from build123d import *

# Parameters (mm, degrees)
F0_R     = 5
F2_DEPTH = 3
F0_R_2   = 1.25
F3_DEPTH = 6
F4_DEPTH = 2


with BuildPart() as f2:
    # F0 (on Top) → F2 (new body)
    with BuildSketch(Plane.XY):
        with BuildLine():
            Line((-6.914658343, 3.5), (-14.0712472795, 3.5))
            ThreePointArc((-14.0712472795, 3.5), (-14.5, 0), (-14.0712472795, -3.5))
            Line((-14.0712472795, -3.5), (-6.914658343, -3.5))
            ThreePointArc((-6.914658343, -3.5), (-7.75, 0), (-6.914658343, 3.5))
        make_face()
        with BuildLine():
            ThreePointArc((7.75, 0), (7.5382724201, 1.7991522784), (6.914658343, 3.5))
            ThreePointArc((6.914658343, 3.5), (0, 7.75), (-6.914658343, 3.5))
            ThreePointArc((-6.914658343, 3.5), (-7.75, 0), (-6.914658343, -3.5))
            ThreePointArc((-6.914658343, -3.5), (0, -7.75), (6.914658343, -3.5))
            ThreePointArc((6.914658343, -3.5), (7.5382724201, -1.7991522784), (7.75, 0))
        make_face()
        Circle(F0_R, mode=Mode.SUBTRACT)
        with BuildLine():
            ThreePointArc((14.0712472795, -3.5), (14.3924126809, -1.7630817405), (14.5, 0))
            ThreePointArc((14.5, 0), (14.3924126809, 1.7630817405), (14.0712472795, 3.5))
            Line((14.0712472795, 3.5), (6.914658343, 3.5))
            ThreePointArc((6.914658343, 3.5), (7.5382724201, 1.7991522784), (7.75, 0))
            ThreePointArc((7.75, 0), (7.5382724201, -1.7991522784), (6.914658343, -3.5))
            Line((6.914658343, -3.5), (14.0712472795, -3.5))
        make_face()
    extrude(amount=F2_DEPTH)

    # F0 (on Top) → F3 (join)
    with BuildSketch(Plane.XY):
        with BuildLine():
            Line((6.914658343, 3.5), (14.0712472795, 3.5))
            ThreePointArc((14.0712472795, 3.5), (0, 14.5), (-14.0712472795, 3.5))
            Line((-14.0712472795, 3.5), (-6.914658343, 3.5))
            ThreePointArc((-6.914658343, 3.5), (0, 7.75), (6.914658343, 3.5))
        make_face()
        with Locations((-7.9549512883, 7.9549512883)):
            Circle(F0_R_2, mode=Mode.SUBTRACT)
        with Locations((7.9549512883, 7.9549512883)):
            Circle(F0_R_2, mode=Mode.SUBTRACT)
        with BuildLine():
            ThreePointArc((-14.0712472795, -3.5), (0, -14.5), (14.0712472795, -3.5))
            Line((14.0712472795, -3.5), (6.914658343, -3.5))
            ThreePointArc((6.914658343, -3.5), (0, -7.75), (-6.914658343, -3.5))
            Line((-6.914658343, -3.5), (-14.0712472795, -3.5))
        make_face()
        with Locations((-7.9549512883, -7.9549512883)):
            Circle(F0_R_2, mode=Mode.SUBTRACT)
        with Locations((7.9549512883, -7.9549512883)):
            Circle(F0_R_2, mode=Mode.SUBTRACT)
    extrude(amount=F3_DEPTH)

    # F0 (on Top) → F4 (join)
    with BuildSketch(Plane.XY):
        Circle(F0_R)
    extrude(amount=F4_DEPTH)


solid = f2.part
Could you check a few things on this model? Use its own coordinates, in mm. A direction names the side the tool comes from. Round coordinates to 2 decimals unless told otherwise and drop trailing zeros. Loops run counter-clockwise (first coordinate to the right, second up) from the corner with the lowest first, then second, coordinate; pieces in that order, holes last. Notation, with made-up numbers: (83.25, 13.25) - (91.25, 13.25) arc R8 ccw to (91.25, 19.25) - close; hole circle Ø11 at (36.25, 42.25). An arc over 180 degrees is marked (long way). Write item = value, one per line.
1) If we mould it in two halves opening along Y, with no side actions, what happens to faces 4 (the cylindrical face through (7.684, 6.735, 2.958)), 5 (the flat face through (0, 9, 6))? For each: pulls with the +Y half, pulls with the -Y half, needs draft (parallel to the pull), parting line crosses it, or undercut.
Computed:
face_4 = undercut
face_5 = needs draft
2) Imagine slicing it at B-B (x = 0). Please give me the cut outline in (y, z).
Computed:
outline = (-14.5, 0) - (14.5, 0) - (14.5, 6) - (7.75, 6) - (7.75, 3) - (5, 3) - (5, 2) - (-5, 2) - (-5, 3) - (-7.75, 3) - (-7.75, 6) - (-14.5, 6) - close
3) On a 3-axis mill with a long thin cutter (end or side, diameter ignored), from which of +Z, -Z, +X, -X, +Y, -Y can I reach the whole of each face in a straight line? I mean faces 1 (the flat face through (11, -3.5, 4)), 2 (the cylindrical face through (-7.378, -9.064, 2.958)), 3 (the cylindrical face through (0.12, -7.75, 4.48)). Say none if no direction works.
Computed:
face_1 = +Z, +X, -X
face_2 = +Z, -Z
face_3 = +Z
4) I need wall thicknesses on line 1 along Y through (x, z) = (12.25, 3.7); line 2 along Y through (x, z) = (0, 2.65); line 3 along X through (y, z) = (4.25, 3.85). Which ranges of each line are inside material? Lowest first, please. Write a range as from..to.
Computed:
line_1 = -7.76..-3.5, 3.5..7.76
line_2 = -14.5..-5, 5..14.5
line_3 = -13.86..-6.48, 6.48..13.86
5) Imagine slicing it at A-A (z = 5.05). Please give me the cut outline in (x, y), and give its area (3 significant figures).
Computed:
outline = (-14.07, -3.5) arc R14.5 ccw to (14.07, -3.5) - (6.91, -3.5) arc R7.75 cw to (-6.91, -3.5) - close; (-14.07, 3.5) - (-6.91, 3.5) arc R7.75 cw to (6.91, 3.5) - (14.07, 3.5) arc R14.5 ccw to start; hole circle Ø2.5 at (-7.95, -7.95); hole circle Ø2.5 at (-7.95, 7.95); hole circle Ø2.5 at (7.95, -7.95); hole circle Ø2.5 at (7.95, 7.95)
area = 356 mm2
6) I'm going to push flat-ended pins straight in: P1, Ø0.9, axis at x = 9.5, z = 5, coming from the +Y side; P2, Ø1.5, axis at x = -7.95, y = -7.95, coming from the -Z side; P3, Ø3, axis at x = 1.5, y = -0.5, coming from the +Z side; P4, Ø3, axis at x = 4, z = 0.5, coming from the -Y side. Where does each tip first touch, or does it pass through?
Computed:
P1 = 11.33
P2 = through
P3 = 2
P4 = -14.28
7) Imagine slicing it at C-C (z = 1.1). Please give me the cut outline in (x, y).
Computed:
outline = circle Ø29 at (0, 0); hole circle Ø2.5 at (-7.95, -7.95); hole circle Ø2.5 at (-7.95, 7.95); hole circle Ø2.5 at (7.95, -7.95); hole circle Ø2.5 at (7.95, 7.95)
8) Imagine slicing it at D-D (y = 1). Please give me the cut outline in (x, z), and give its area (3 significant figures).
Computed:
outline = (-14.47, 0) - (14.47, 0) - (14.47, 3) - (4.9, 3) - (4.9, 2) - (-4.9, 2) - (-4.9, 3) - (-14.47, 3) - close
area = 77.0 mm2
